The figure shows three views and two pictorial views of one solid part (mm, origin at its lowest corner). Answer the questions. Give positions to 0.01 mm unless a question says otherwise; leave off trailing zeros. Write each loop counter-clockwise with the first axis right and the second up, starting at its lowest first coordinate (ties: lowest second). Pieces come first, ordered by that corner, then holes. Notation, with made-up numbers: M 48.5,14.5 L 89.5,14.5 A29 ccw 89.5,34.5 Z; hole C 88.5,-20.5 d8. An arc over 180 degrees is marked long. Return JSON: item names as keys, results as strings.
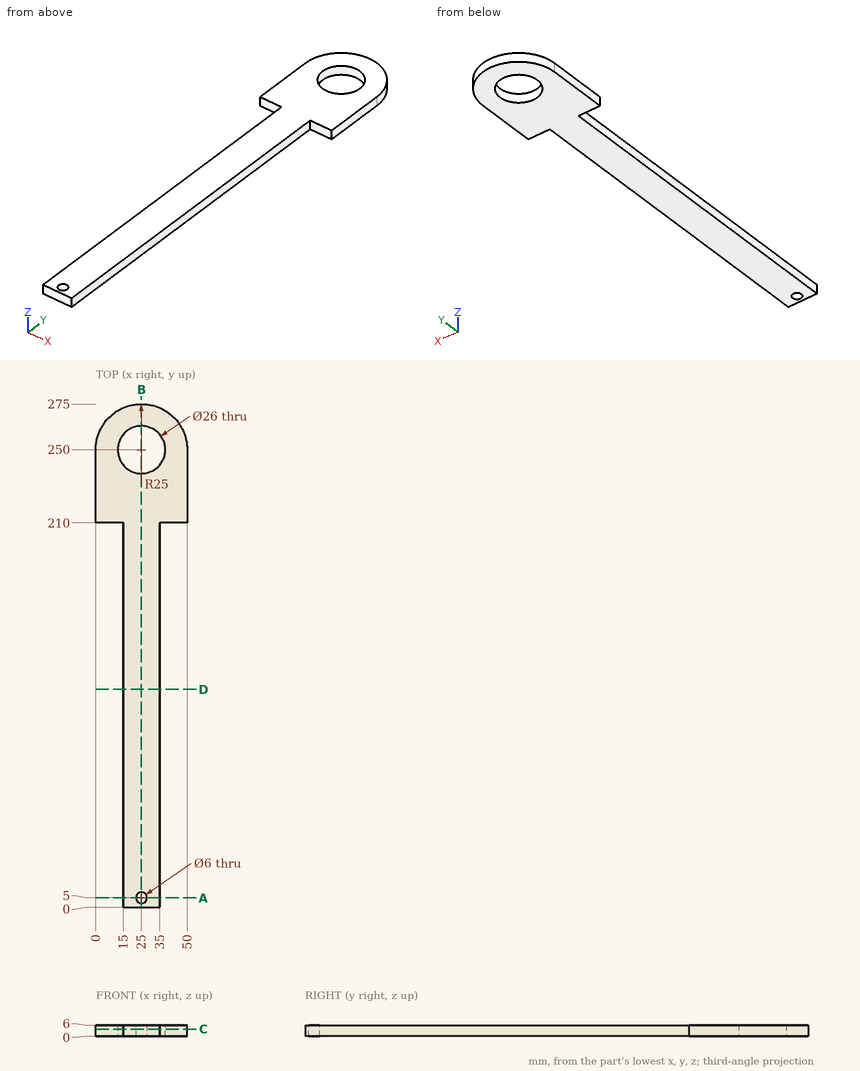
Item 1: Find the intervals of material crossed by line 1 (Y direction, x = 25, z = 1.9); line 2 (Y direction, x = 26, z = 5.45); line 3 (X direction, y = 5, z = 3.65), in increasing order.
Geometry results:
{"line 1": "y = 0 to 2, 8 to 237, 263 to 275", "line 2": "y = 0 to 2.17, 7.83 to 237.04, 262.96 to 274.98", "line 3": "x = 15 to 22, 28 to 35"}
Item 2: A cutting plane is placed at C-C, the plane z = 3.7. Write down the section's boundary in (x, y), plus the area to 3 significant figures.
Geometry results:
{"outline": "M 0,210 L 15,210 L 15,0 L 35,0 L 35,210 L 50,210 L 50,250 A25 ccw 0,250 Z; hole C 25,250 d26; hole C 25,5 d6", "area": "6,620 mm2"}
Item 3: A cutting plane is placed at B-B, the plane x = 25. Write down the section's boundary in (y, z), plus the area to 3 significant figures.
Geometry results:
{"outline": "M 0,0 L 2,0 L 2,6 L 0,6 Z; M 8,0 L 237,0 L 237,6 L 8,6 Z; M 263,0 L 275,0 L 275,6 L 263,6 Z", "area": "1,460 mm2"}
Item 4: A cutting plane is placed at A-A, the plane y = 5. Write down the section's boundary in (x, z).
Geometry results:
{"outline": "M 15,0 L 22,0 L 22,6 L 15,6 Z; M 28,0 L 35,0 L 35,6 L 28,6 Z"}
Item 5: A cutting plane is placed at D-D, the plane y = 119. Write down the section's boundary in (x, z).
Geometry results:
{"outline": "M 15,0 L 35,0 L 35,6 L 15,6 Z"}
Item 6: Given pin 1 Ø2 at (y, z) = (166, 2.5) entering from -X; pin 2 Ø1.8 at (y, z) = (75, 4) entering from +X; pin 3 Ø1 at (x, z) = (43.5, 5) entering from -Y, each flat-ended and moving along its own axis, determine where each tip first touches the part or whether it passes through.
Geometry results:
{"pin 1": "stops at x = 15", "pin 2": "stops at x = 35", "pin 3": "stops at y = 210"}
